Part print with two shaded views. Sizes in mm from the minimum x, y, z corner. Give positions to 0.01 mm unless a question says otherwise; leave off trailing zeros. Write each loop counter-clockwise with the first axis right and the second up, starting at its lowest first coordinate (ties: lowest second). Pieces come first, ordered by that corner, then holes. Notation, with made-up numbers: M 28,-30.5 L 56,-30.5 A13 cw 56,-18.5 Z; hole C -12,58.5 d7. An arc over 180 degrees is marked long. Return JSON: item names as keys, results as strings. Group by question number.
Q1. Band-saw the part on A-A, the plane x = 25. Give the cut face in (y, z), then the cut area to 3 significant figures.
Q2. Wall check: probe 1 along Y at (x, z) = (25, 6.6); probe 2 along Y at (x, z) = (25, 1.8). Give the ranges that are in metal, low to high.
Q3. Band-saw the part on C-C, the plane z = 7. Give the cut face in (x, y), then the cut area to 3 significant figures.
Q4. Flat gauge pin, fed straight in: pin 1 Ø5.5 at (x, y) = (25, 25) entering from +Z. Where does the tip first touch, or does it go through?
Q5. Pull direction X, two halves, no side cores. Call the marked faces 1, 2, 3 and 4: +X half, -X half, draft (parallel to the pull), parting line (faces both ways), or undercut.
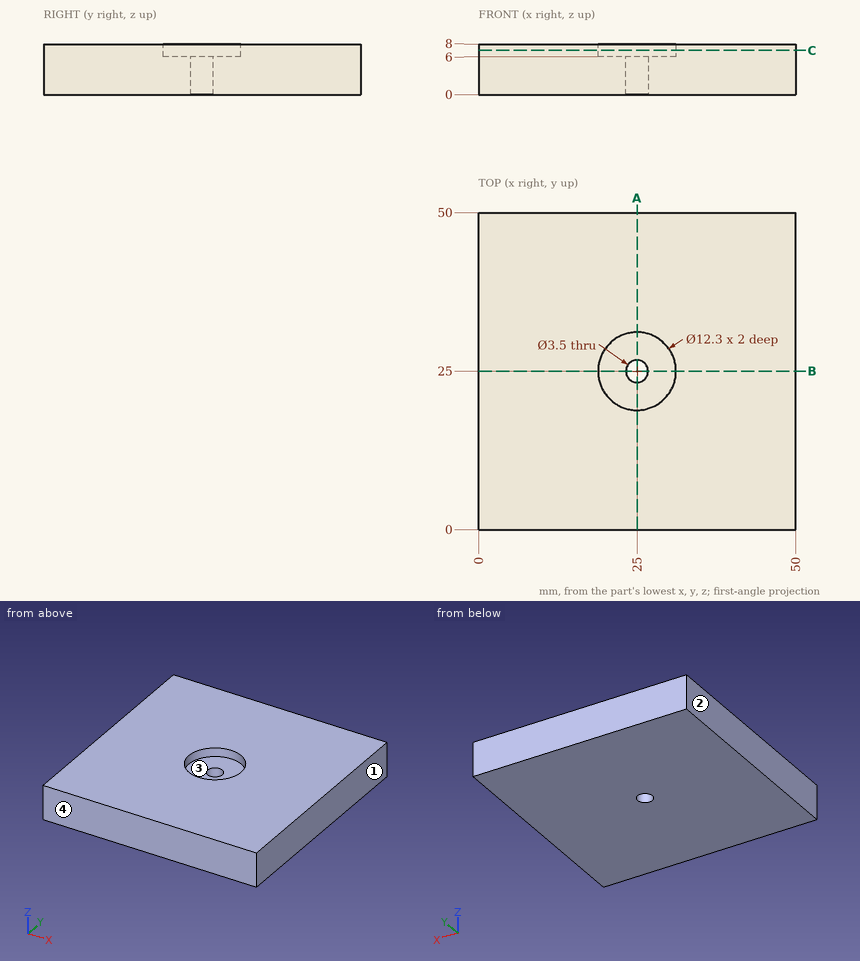
From the geometry:
{
 "1": {"outline": "M 0,0 L 23.25,0 L 23.25,6 L 18.85,6 L 18.85,8 L 0,8 Z; M 26.75,0 L 50,0 L 50,8 L 31.15,8 L 31.15,6 L 26.75,6 Z", "area": "354 mm^2"},
 "2": {"probe 1": "y = 0 to 18.85, 31.15 to 50", "probe 2": "y = 0 to 23.25, 26.75 to 50"},
 "3": {"outline": "M 0,0 L 50,0 L 50,50 L 0,50 Z; hole C 25,25 d12.3", "area": "2,380 mm^2"},
 "4": {"pin 1": "stops at z = 6"},
 "5": {"face 1": "+X half", "face 2": "-X half", "face 3": "undercut", "face 4": "draft"}
}
